```python
from build123d import *

# Parameters (mm, degrees)
BOSS_EXTRUDE1_DEPTH            = 17
SKETCH2_W                      = 41.219755562
SKETCH2_H                      = 3.074219812
CUT_EXTRUDE1_DEPTH             = 84.08770607
SKETCH3_W                      = 41.219755562
SKETCH3_H                      = 1.5
CUT_EXTRUDE2_DEPTH             = 84.08770607
BOSS_EXTRUDE2_DEPTH            = 3
BOSS_EXTRUDE3_DEPTH            = 3
SKETCH6_W                      = 31.19276455
SKETCH6_H                      = 12
BOSS_EXTRUDE4_DEPTH            = 19.5
SKETCH7_W                      = 31.19276455
SKETCH7_H                      = 12
BOSS_EXTRUDE5_DEPTH            = 19.5
DRAFT1_ANGLE                   = 5.033187306
DRAFT2_ANGLE                   = 5.033187306
F_4_1_4_1_DIAMETER_HOLE1_D     = 4.1
F_4_1_4_1_DIAMETER_HOLE1_DEPTH = 5
F_4_0_4_DIAMETER_HOLE1_D       = 4
F_4_0_4_DIAMETER_HOLE1_DEPTH   = 16
F_8_0_8_DIAMETER_HOLE1_D       = 8
F_8_0_8_DIAMETER_HOLE1_DEPTH   = 20


with BuildPart() as part:
    # Sketch1 → Boss-Extrude1 (new body)
    with BuildSketch(Plane(origin=(0, 13, 0), x_dir=(1, 0, 0), z_dir=(0, 1, 0))):
        Polygon((-26.080793056, -23.37), (26.080793056, -23.37), (77.9, -18.806160436), (77.9, 18.806160436), (26.080793056, 23.37), (-26.080793056, 23.37), (-77.9, 18.806160436), (-77.9, -18.806160436), align=None)
    extrude(amount=-BOSS_EXTRUDE1_DEPTH)

    # Sketch2 → Cut-Extrude1 (cut, through all)
    with BuildSketch(Plane.XZ.offset(4)):
        with Locations((0, 21.832890094)):
            Rectangle(SKETCH2_W, SKETCH2_H)
    extrude(amount=-CUT_EXTRUDE1_DEPTH, mode=Mode.SUBTRACT)

    # Sketch3 → Cut-Extrude2 (cut, through all)
    with BuildSketch(Plane.XZ.offset(4)):
        with Locations((0, -22.62)):
            Rectangle(SKETCH3_W, SKETCH3_H)
    extrude(amount=-CUT_EXTRUDE2_DEPTH, mode=Mode.SUBTRACT)

    # Sketch4 → Boss-Extrude2 (add)
    with BuildSketch(Plane(origin=(0, 13, 0), x_dir=(-1, 0, 0), z_dir=(0, 1, 0))):
        Polygon((-20.609877781, 20.295780188), (-20.609877781, 23.37), (-26.080793056, 23.37), (-77.9, 18.806160436), (-77.9, -18.806160436), (-26.080793056, -23.37), (-20.609877781, -23.37), (-20.609877781, -21.87), align=None)
    extrude(amount=BOSS_EXTRUDE2_DEPTH)

    # Sketch5 → Boss-Extrude3 (add)
    with BuildSketch(Plane(origin=(0, 13, 0), x_dir=(-1, 0, 0), z_dir=(0, 1, 0))):
        Polygon((20.609877781, -21.87), (20.609877781, -23.37), (26.080793056, -23.37), (77.9, -18.806160436), (77.9, 18.806160436), (26.080793056, 23.37), (20.609877781, 23.37), (20.609877781, 20.295780188), align=None)
    extrude(amount=BOSS_EXTRUDE3_DEPTH)

    # Sketch6 → Boss-Extrude4 (add)
    with BuildSketch(Plane(origin=(77.9, 0, 0), x_dir=(0, 0, -1), z_dir=(1, 0, 0))):
        with Locations((0, 6)):
            Rectangle(SKETCH6_W, SKETCH6_H)
    extrude(amount=BOSS_EXTRUDE4_DEPTH)

    # Sketch7 → Boss-Extrude5 (add)
    with BuildSketch(Plane.ZY.offset(77.9)):
        with Locations((0, 6)):
            Rectangle(SKETCH7_W, SKETCH7_H)
    extrude(amount=BOSS_EXTRUDE5_DEPTH)

    # Draft1
    draft1_faces = [part.faces().sort_by_distance(p)[0] for p in [
        (-87.65, 6, 15.596382275),
        (-87.65, 6, -15.596382275),
    ]]
    draft(draft1_faces, Plane(origin=(-77.9, -4, -18.806160436), x_dir=(0, 0, -1), z_dir=(-1, 0, 0)), DRAFT1_ANGLE)

    # Draft2
    draft2_faces = [part.faces().sort_by_distance(p)[0] for p in [
        (87.65, 6, 15.596382275),
        (87.65, 6, -15.596382275),
    ]]
    draft(draft2_faces, Plane(origin=(77.9, -4, 18.806160436), x_dir=(0, 0, 1), z_dir=(1, 0, 0)), DRAFT2_ANGLE)

    # Ø4.1 (4.1) Diameter Hole1
    with Locations(Plane.XY.offset(23.37)):
        with Locations((-10, 4.5), (10, 4.5)):
            Hole(F_4_1_4_1_DIAMETER_HOLE1_D / 2, depth=F_4_1_4_1_DIAMETER_HOLE1_DEPTH)

    # Ø4.0 (4) Diameter Hole1
    with Locations(Plane(origin=(0, 12, 0), x_dir=(1, 0, 0), z_dir=(0, 1, 0))):
        with Locations((-83, 6), (-83, -6), (83, -6), (83, 6)):
            Hole(F_4_0_4_DIAMETER_HOLE1_D / 2, depth=F_4_0_4_DIAMETER_HOLE1_DEPTH)

    # Ø8.0 (8) Diameter Hole1
    with Locations(Plane(origin=(0, -4, 0), x_dir=(-1, 0, 0), z_dir=(0, -1, 0))):
        with Locations((0, 0)):
            Hole(F_8_0_8_DIAMETER_HOLE1_D / 2, depth=F_8_0_8_DIAMETER_HOLE1_DEPTH)


solid = part.part
```
The model under review builds one solid part; all positions refer to its coordinate system, in mm. A direction names the side the tool comes from. Coordinates: 2 decimals unless noted, no trailing zeros. Write each loop counter-clockwise with the first axis right and the second up, starting at its lowest first coordinate (ties: lowest second). Pieces come first, ordered by that corner, then holes.
1) We need section A-A on y = 8.25. Count the separate pieces of the cut face and the enclosed holes in it, then the cut area to 3 significant figures.
2) To check wall thickness, follow probe 1 along Z at (x, y) = (-83, 4); probe 2 along Y at (x, z) = (10, 18.8); probe 3 along Z at (x, y) = (0, 7.5). State the ranges of each line that lie inside material, in increasing order.
3) Machinability: for faces 1 (the face through (88, 12, 0)), 2 (the face through (-20.61, 14, 4)), 3 (the face through (-51.63, 5.86, -21.12)), 4 (the face through (0, 4, 20.296)), which of the approach directions +Z, -Z, +X, -X, +Y, -Y give a long, thin tool a straight path to every point of the face, cutting with its end or side? Answer none if there is none.
4) We need section C-C on x = -10. State the section outline as (y, z) points, then the cut area to 3 significant figures.
5) Clearance check with flat-ended pins moving along their axes: pin 1 Ø6.5 at (x, z) = (-83, 6) entering from -Y; pin 2 Ø3.5 at (x, y) = (9, 4.5) entering from +Z; pin 3 Ø2 at (x, y) = (66, 6) entering from +Z; pin 4 Ø3.5 at (x, z) = (-83, -6) entering from -Y. State where each tip first meets the part, or that it passes through.
6) We need section D-D on z = -10. State the section outline as (x, y) points.
7) The part is to be moulded in two halves that separate along Z. For faces 5 (the face through (97.4, 6, 0)), 6 (the face through (52.353, 5.86, -21.056)), 7 (the face through (-87.51, 5.92, 14.75)), 8 (the face through (81.092, 5.916, -6.601)), say which applies: pulls with the +Z half, pulls with the -Z half, needs draft (parallel to the pull), parting line crosses it, or undercut.
8) We need section B-B on z = 0. State the section outline as (x, y) points.
Answer list:
1. separate pieces: 1
1. enclosed holes: 5
1. area: 7,670 mm2
2. probe 1: z = -15.15 to -8, -4 to 4, 8 to 15.15
2. probe 2: y = -4 to 2.45, 6.55 to 13
2. probe 3: z = -21.87 to -4, 4 to 20.3
3. face 1: +Z, -Z, +X, +Y
3. face 2: +Y
3. face 3: -Z, -X, +Y, -Y
3. face 4: +Z, +Y, -Y
4. outline: (-4, -21.87) - (13, -21.87) - (13, 20.3) - (6.55, 20.3) - (6.55, 18.37) - (2.45, 18.37) - (2.45, 20.3) - (-4, 20.3) - close
4. area: 709 mm2
5. pin 1: stops at y = 0
5. pin 2: stops at z = 20.3
5. pin 3: stops at z = 19.94
5. pin 4: passes through
6. outline: (-97.4, 0) - (-77.9, 0) - (-77.9, -4) - (77.9, -4) - (77.9, 0) - (97.4, 0) - (97.4, 12) - (77.9, 12) - (77.9, 16) - (20.61, 16) - (20.61, 13) - (-20.61, 13) - (-20.61, 16) - (-77.9, 16) - (-77.9, 12) - (-97.4, 12) - close
7. face 5: needs draft
7. face 6: pulls with the -Z half
7. face 7: pulls with the +Z half
7. face 8: undercut
8. outline: (-97.4, 0) - (-77.9, 0) - (-77.9, -4) - (-4, -4) - (-4, 13) - (-20.61, 13) - (-20.61, 16) - (-77.9, 16) - (-77.9, 12) - (-97.4, 12) - close; (4, -4) - (77.9, -4) - (77.9, 0) - (97.4, 0) - (97.4, 12) - (77.9, 12) - (77.9, 16) - (20.61, 16) - (20.61, 13) - (4, 13) - close
